The model under review builds one solid part; all positions refer to its coordinate system, in mm. Face numbers are marked on the shaded views. A direction names the side the tool comes from. Coordinates: 2 decimals unless noted, no trailing zeros. Write each loop counter-clockwise with the first axis right and the second up, starting at its lowest first coordinate (ties: lowest second). Pieces come first, ordered by that corner, then holes.
1) For line 1 (X direction, y = 1.6, z = -14); line 2 (X direction, y = 71, z = 22.5); line 3 (Z direction, x = 30.3, y = 69.25), list the stretches that pass through material, from the lowest coordinate up.
2) Mouldability with a two-part tool opening along X and no side actions: class the marked faces 3, 4 and 5 as released by +X, released by -X, zero draft, split by the parting line, or undercut.
3) Add section D-D, the plane y = 69.25. State the section outline as (x, z) points, then the cut area to 3 significant figures.
4) Add section B-B, the plane x = 14. State the section outline as (y, z) points.
5) For P1, Ø2, axis at x = 9, z = -13, coming from the -Y side; P2, Ø4.5, axis at x = -14, z = -14, coming from the +Y side, all flat-tipped, find the tip position at first contact; note any pin that passes through.
6) Machinability: for the marked faces 1 and 2, which of the approach directions +Z, -Z, +X, -X, +Y, -Y give a long, thin tool a straight path to every point of the face, cutting with its end or side? Answer none if there is none.
7) Add section A-A, the plane y = 49. State the section outline as (x, z) points, then the cut area to 3 significant figures.
8) Add section C-C, the plane z = -14. State the section outline as (x, y) points.
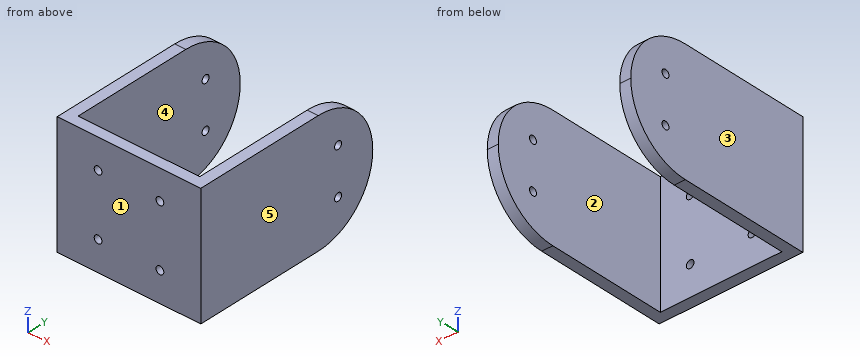
from build123d import *

# Parameters (mm, degrees)
SKETCH1_W              = 65
SKETCH1_H              = 55
BOSS_EXTRUDE1_DEPTH    = 5
SKETCH2_W              = 5
SKETCH2_H              = 55
BOSS_EXTRUDE2_DEPTH    = 81.75
CUT_EXTRUDE1_START     = -5
CUT_EXTRUDE1_OUTLINE_R = 1.75
CUT_EXTRUDE1_DEPTH     = 5
CUT_EXTRUDE2_REACH     = 98.634
SKETCH4_R              = 1.75


# Read off the part's stored shape, not the designer's step: Cut-Extrude1
with BuildPart() as part:
    # Sketch1 → Boss-Extrude1 (new body)
    with BuildSketch(Plane(origin=(0, 0, 0), x_dir=(1, 0, 0), z_dir=(0, 1, 0))):
        Rectangle(SKETCH1_W, SKETCH1_H)
    extrude(amount=BOSS_EXTRUDE1_DEPTH)

    # Sketch2 → Boss-Extrude2 (add)
    with BuildSketch(Plane(origin=(0, 5, 0), x_dir=(1, 0, 0), z_dir=(0, 1, 0))):
        with Locations((-30, 0)):
            Rectangle(SKETCH2_W, SKETCH2_H)
        with Locations((30, 0)):
            Rectangle(SKETCH2_W, SKETCH2_H)
    extrude(amount=BOSS_EXTRUDE2_DEPTH)

    # Cut-Extrude1 outline → Cut-Extrude1 (cut)
    with BuildSketch(Plane.ZY.offset(32.5).offset(CUT_EXTRUDE1_START)):
        with BuildLine():
            ThreePointArc((-27.5, 59.25), (-19.445436473, 78.695436492), (2.6e-08, 86.75))
            Line((2.6e-08, 86.75), (-27.5, 86.75))
            Line((-27.5, 86.75), (-27.5, 59.25))
        make_face()
        with BuildLine():
            ThreePointArc((2.6e-08, 86.75), (19.445436492, 78.695436473), (27.5, 59.25))
            Line((27.5, 59.25), (27.5, 86.75))
            Line((27.5, 86.75), (2.6e-08, 86.75))
        make_face()
        with Locations((-10.5, 69.25)):
            Circle(CUT_EXTRUDE1_OUTLINE_R)
        with Locations((10.5, 69.25)):
            Circle(CUT_EXTRUDE1_OUTLINE_R)
    cut_extrude1 = extrude(amount=CUT_EXTRUDE1_DEPTH, mode=Mode.SUBTRACT)

    # Mirror1: Cut-Extrude1 across plane
    add(cut_extrude1.mirror(Plane(origin=(0, 0, 0), x_dir=(0, 0, 1), z_dir=(1, 0, 0))), mode=Mode.SUBTRACT)

    # Sketch4 → Cut-Extrude2 (cut, up to next)
    with BuildSketch(Plane.XZ, mode=Mode.PRIVATE) as cut_extrude2_sk1:
        with Locations(Location((-14, 14, 0), (0, 0, 270))):
            Circle(SKETCH4_R)
    cut_extrude2_tool1 = extrude(cut_extrude2_sk1.sketch, amount=-CUT_EXTRUDE2_REACH, mode=Mode.PRIVATE) & part.part
    # Sketch4 → Cut-Extrude2 (cut, up to next)
    with BuildSketch(Plane.XZ, mode=Mode.PRIVATE) as cut_extrude2_sk2:
        with Locations(Location((-14, -14, 0), (0, 0, 270))):
            Circle(SKETCH4_R)
    cut_extrude2_tool2 = extrude(cut_extrude2_sk2.sketch, amount=-CUT_EXTRUDE2_REACH, mode=Mode.PRIVATE) & part.part
    # Sketch4 → Cut-Extrude2 (cut, up to next)
    with BuildSketch(Plane.XZ, mode=Mode.PRIVATE) as cut_extrude2_sk3:
        with Locations(Location((14, -14, 0), (0, 0, 270))):
            Circle(SKETCH4_R)
    cut_extrude2_tool3 = extrude(cut_extrude2_sk3.sketch, amount=-CUT_EXTRUDE2_REACH, mode=Mode.PRIVATE) & part.part
    # Sketch4 → Cut-Extrude2 (cut, up to next)
    with BuildSketch(Plane.XZ, mode=Mode.PRIVATE) as cut_extrude2_sk4:
        with Locations(Location((14, 14, 0), (0, 0, 270))):
            Circle(SKETCH4_R)
    cut_extrude2_tool4 = extrude(cut_extrude2_sk4.sketch, amount=-CUT_EXTRUDE2_REACH, mode=Mode.PRIVATE) & part.part
    add(cut_extrude2_tool1.solids().sort_by_distance((-14, 0, 14))[0], mode=Mode.SUBTRACT)
    add(cut_extrude2_tool2.solids().sort_by_distance((-14, 0, -14))[0], mode=Mode.SUBTRACT)
    add(cut_extrude2_tool3.solids().sort_by_distance((14, 0, -14))[0], mode=Mode.SUBTRACT)
    add(cut_extrude2_tool4.solids().sort_by_distance((14, 0, 14))[0], mode=Mode.SUBTRACT)


solid = part.part
Geometry results:
1. line 1: x = -32.5 to -15.75, -12.25 to 12.25, 15.75 to 32.5
1. line 2: x = -32.5 to -27.5, 27.5 to 32.5
1. line 3: z = -25.62 to -12.25, -8.75 to 8.75, 12.25 to 25.62
2. face 3: released by -X
2. face 4: undercut
2. face 5: released by +X
3. outline: (-32.5, -25.62) - (-27.5, -25.62) - (-27.5, -12.25) - (-32.5, -12.25) - close; (-32.5, -8.75) - (-27.5, -8.75) - (-27.5, 8.75) - (-32.5, 8.75) - close; (-32.5, 12.25) - (-27.5, 12.25) - (-27.5, 25.62) - (-32.5, 25.62) - close; (27.5, -25.62) - (32.5, -25.62) - (32.5, -12.25) - (27.5, -12.25) - close; (27.5, -8.75) - (32.5, -8.75) - (32.5, 8.75) - (27.5, 8.75) - close; (27.5, 12.25) - (32.5, 12.25) - (32.5, 25.62) - (27.5, 25.62) - close
3. area: 442 mm2
4. outline: (0, -27.5) - (5, -27.5) - (5, -15.75) - (0, -15.75) - close; (0, -12.25) - (5, -12.25) - (5, 12.25) - (0, 12.25) - close; (0, 15.75) - (5, 15.75) - (5, 27.5) - (0, 27.5) - close
5. P1: stops at y = 0
5. P2: stops at y = 5
6. face 1: +Z, -Z, +X, -X, -Y
6. face 2: +Z, -Z, +Y
7. outline: (-32.5, -27.5) - (-27.5, -27.5) - (-27.5, 27.5) - (-32.5, 27.5) - close; (27.5, -27.5) - (32.5, -27.5) - (32.5, 27.5) - (27.5, 27.5) - close
7. area: 550 mm2
8. outline: (-32.5, 0) - (-15.75, 0) - (-15.75, 5) - (-27.5, 5) - (-27.5, 82.92) - (-32.5, 82.92) - close; (-12.25, 0) - (12.25, 0) - (12.25, 5) - (-12.25, 5) - close; (15.75, 0) - (32.5, 0) - (32.5, 82.92) - (27.5, 82.92) - (27.5, 5) - (15.75, 5) - close
